The listing builds one solid part. Answer for the finished solid, in the listing's coordinates (mm). Face numbers are marked on the shaded views. Give positions to 0.01 mm unless a question says otherwise; leave off trailing zeros. Write each loop counter-clockwise with the first axis right and the second up, starting at its lowest first coordinate (ties: lowest second). Pieces come first, ordered by that corner, then holes. Notation, with made-up numbers: (-3, 35) - (48, 35) arc R34 cw to (48, 69) - close; hole circle Ø6 at (54, 33). An arc over 180 degrees is marked (long way). Use a Markdown table: item, result. Add a question column.
from build123d import *

# Parameters (mm, degrees)
BOSS_EXTRUDE1_DEPTH     = 6.5
SKETCH2_R               = 27.5
BOSS_EXTRUDE2_DEPTH     = 2.5
CUT_EXTRUDE1_DEPTH      = 8
SKETCH4_W               = 3
SKETCH4_H               = 3
CUT_EXTRUDE2_DEPTH      = 10
SKETCH5_R               = 5
BOSS_EXTRUDE3_DEPTH     = 140
CUT_EXTRUDE3_DEPTH      = 15
MIRROR6_COPY_1_SKETCH_R = 27.5
MIRROR6_COPY_1_DEPTH    = 2.5
MIRROR6_COPY_2_SKETCH_W = 3
MIRROR6_COPY_2_SKETCH_H = 3
MIRROR6_COPY_2_DEPTH    = 10


with BuildPart() as part:
    # Sketch1 → Boss-Extrude1 (new body)
    with BuildSketch(Plane(origin=(0, 0, 0), x_dir=(1, 0, 0), z_dir=(0, 1, 0))):
        with BuildLine():
            ThreePointArc((-1.9, -2.05669638), (-2.8, 0), (-1.9, 2.05669638))
            Line((-1.9, 2.05669638), (-1.9, 5.532856405))
            ThreePointArc((-1.9, 5.532856405), (-5.85, 0), (-1.9, -5.532856405))
            Line((-1.9, -5.532856405), (-1.9, -2.05669638))
        make_face()
        with BuildLine():
            ThreePointArc((-1.9, 2.05669638), (0, 2.8), (1.9, 2.05669638))
            Line((1.9, 2.05669638), (1.9, 5.532856405))
            ThreePointArc((1.9, 5.532856405), (0, 5.85), (-1.9, 5.532856405))
            Line((-1.9, 5.532856405), (-1.9, 2.05669638))
        make_face()
        with BuildLine():
            Line((1.9, 5.532856405), (1.9, 2.05669638))
            ThreePointArc((1.9, 2.05669638), (2.565151068, 1.122497216), (2.8, 0))
            ThreePointArc((2.8, 0), (2.565151068, -1.122497216), (1.9, -2.05669638))
            Line((1.9, -2.05669638), (1.9, -5.532856405))
            ThreePointArc((1.9, -5.532856405), (4.761171074, -3.399080758), (5.85, 0))
            ThreePointArc((5.85, 0), (4.761171074, 3.399080758), (1.9, 5.532856405))
        make_face()
        with BuildLine():
            Line((1.9, -5.532856405), (1.9, -2.05669638))
            ThreePointArc((1.9, -2.05669638), (0, -2.8), (-1.9, -2.05669638))
            Line((-1.9, -2.05669638), (-1.9, -5.532856405))
            ThreePointArc((-1.9, -5.532856405), (0, -5.85), (1.9, -5.532856405))
        make_face()
        with BuildLine():
            Line((-1.9, -2.05669638), (-1.9, 2.05669638))
            ThreePointArc((-1.9, 2.05669638), (-2.8, 0), (-1.9, -2.05669638))
        make_face()
        with BuildLine():
            ThreePointArc((2.8, 0), (2.565151068, 1.122497216), (1.9, 2.05669638))
            Line((1.9, 2.05669638), (1.9, -2.05669638))
            ThreePointArc((1.9, -2.05669638), (2.565151068, -1.122497216), (2.8, 0))
        make_face()
    boss_extrude1 = extrude(amount=BOSS_EXTRUDE1_DEPTH)

    # Sketch2 → Boss-Extrude2 (add)
    with BuildSketch(Plane(origin=(0, 6.5, 0), x_dir=(1, 0, 0), z_dir=(0, 1, 0))):
        with Locations(Location((0, 0, 0), (0, 0, 270))):
            Circle(SKETCH2_R)
    boss_extrude2 = extrude(amount=-BOSS_EXTRUDE2_DEPTH)

    # Sketch3 → Cut-Extrude1 (cut)
    with BuildSketch(Plane.XZ.offset(-4)):
        with BuildLine():
            Line((-1.9, 2.05669638), (-1.9, -2.05669638))
            ThreePointArc((-1.9, -2.05669638), (0, -2.8), (1.9, -2.05669638))
            Line((1.9, -2.05669638), (1.9, 2.05669638))
            ThreePointArc((1.9, 2.05669638), (0, 2.8), (-1.9, 2.05669638))
        make_face()
    cut_extrude1 = extrude(amount=-CUT_EXTRUDE1_DEPTH, mode=Mode.SUBTRACT)

    # Sketch4 → Cut-Extrude2 (cut)
    with BuildSketch(Plane(origin=(0, 6.5, 0), x_dir=(1, 0, 0), z_dir=(0, 1, 0))):
        Polygon((14.299038106, -21.766660498), (15.799038106, -24.36473671), (13.200961894, -25.86473671), (11.700961894, -23.266660498), align=None)
        with Locations((27.5, 0)):
            Rectangle(SKETCH4_W, SKETCH4_H)
        Polygon((-11.700961894, -23.266660498), (-13.200961894, -25.86473671), (-15.799038106, -24.36473671), (-14.299038106, -21.766660498), align=None)
        with Locations((-27.5, 0)):
            Rectangle(SKETCH4_W, SKETCH4_H)
        Polygon((-14.299038106, 21.766660498), (-15.799038106, 24.36473671), (-13.200961894, 25.86473671), (-11.700961894, 23.266660498), align=None)
        Polygon((11.700961894, 23.266660498), (13.200961894, 25.86473671), (15.799038106, 24.36473671), (14.299038106, 21.766660498), align=None)
    cut_extrude2 = extrude(amount=-CUT_EXTRUDE2_DEPTH, mode=Mode.SUBTRACT)

    # Sketch5 → Boss-Extrude3 (add)
    with BuildSketch(Plane(origin=(0, 6.5, 0), x_dir=(1, 0, 0), z_dir=(0, 1, 0))):
        with Locations(Location((0, 0, 0), (0, 0, 270))):
            Circle(SKETCH5_R)
    extrude(amount=BOSS_EXTRUDE3_DEPTH)

    # Mirror1: Boss-Extrude2 across plane
    add(boss_extrude2.mirror(Plane.ZX.offset(76.5)))

    # Mirror2: Boss-Extrude1 across plane
    add(boss_extrude1.mirror(Plane.ZX.offset(76.5)))

    # Mirror3: Boss-Extrude2, Cut-Extrude1, Cut-Extrude2 across plane
    add(boss_extrude2.mirror(Plane.ZX.offset(7.5)))
    add(cut_extrude1.mirror(Plane.ZX.offset(7.5)), mode=Mode.SUBTRACT)
    add(cut_extrude2.mirror(Plane.ZX.offset(7.5)), mode=Mode.SUBTRACT)

    # Sketch6 → Cut-Extrude3 (cut)
    with BuildSketch(Plane.XZ.offset(-11)):
        with BuildLine():
            Line((-1.9, 2.05669638), (-1.9, -2.05669638))
            ThreePointArc((-1.9, -2.05669638), (0, -2.8), (1.9, -2.05669638))
            Line((1.9, -2.05669638), (1.9, 2.05669638))
            ThreePointArc((1.9, 2.05669638), (0, 2.8), (-1.9, 2.05669638))
        make_face()
    extrude(amount=-CUT_EXTRUDE3_DEPTH, mode=Mode.SUBTRACT)

    # Mirror5: Cut-Extrude2 across plane
    add(cut_extrude2.mirror(Plane.ZX.offset(76.5)), mode=Mode.SUBTRACT)

    # Mirror6 copy 1 sketch → Mirror6 copy 1 (add)
    with BuildSketch(Plane(origin=(0, 144.5, 0), x_dir=(1, 0, 0), z_dir=(0, 1, 0))):
        with Locations(Location((0, 0, 0), (0, 0, 270))):
            Circle(MIRROR6_COPY_1_SKETCH_R)
    extrude(amount=-MIRROR6_COPY_1_DEPTH)

    # Mirror6 copy 2 sketch → Mirror6 copy 2 (cut)
    with BuildSketch(Plane(origin=(0, 144.5, 0), x_dir=(1, 0, 0), z_dir=(0, 1, 0))):
        Polygon((14.299038106, -21.766660498), (15.799038106, -24.36473671), (13.200961894, -25.86473671), (11.700961894, -23.266660498), align=None)
        with Locations((27.5, 0)):
            Rectangle(MIRROR6_COPY_2_SKETCH_W, MIRROR6_COPY_2_SKETCH_H)
        Polygon((-11.700961894, -23.266660498), (-13.200961894, -25.86473671), (-15.799038106, -24.36473671), (-14.299038106, -21.766660498), align=None)
        with Locations((-27.5, 0)):
            Rectangle(MIRROR6_COPY_2_SKETCH_W, MIRROR6_COPY_2_SKETCH_H)
        Polygon((-14.299038106, 21.766660498), (-15.799038106, 24.36473671), (-13.200961894, 25.86473671), (-11.700961894, 23.266660498), align=None)
        Polygon((11.700961894, 23.266660498), (13.200961894, 25.86473671), (15.799038106, 24.36473671), (14.299038106, 21.766660498), align=None)
    extrude(amount=-MIRROR6_COPY_2_DEPTH, mode=Mode.SUBTRACT)


solid = part.part
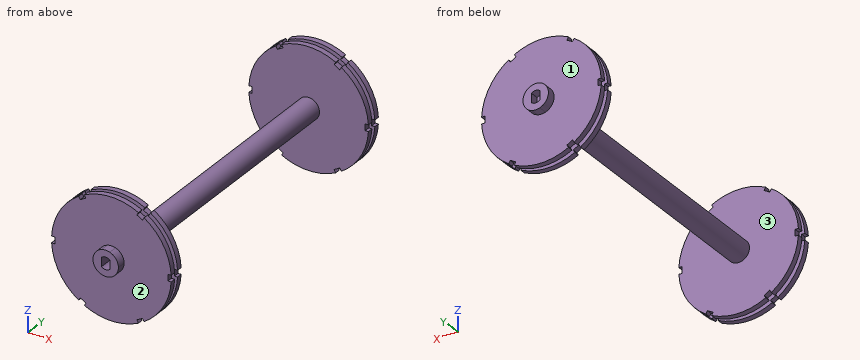
1. The part is cut by section B-B (x = 19). Give the vertices of the cut face in (y, z), and give its area (3 significant figures).
2. Given P1, Ø5, axis at y = 106, z = 6, coming from the +X side; P2, Ø5, axis at x = -5, y = 32, coming from the -Z side; P3, Ø10, axis at y = 136.5, z = 8, coming from the +X side; P4, Ø2, axis at y = 70, z = -7.5, coming from the -X side (1 decimal), each flat-ended and moving along its own axis, determine where each tip first touches the part or whether it passes through.
3. The part is cut by section A-A (z = 9). Give the vertices of the cut face in (x, y), and give its area (3 significant figures).
4. For a pull along Y with two mould halves and no side action, classify the marked faces 1, 2 and 3 as released by +Y, released by -Y, zero draft, split by the parting line, or undercut.
5. The part is cut by section C-C (y = 123). Give the vertices of the cut face in (x, z).
6. Consider L1, parallel to Y at x = 15, z = -20; L2, parallel to X at y = 93, z = -0.5; L3, parallel to X at y = 17, z = 1. Determine where each line is inside the solid, lowest interval first. Write a range as [from, to].
Check values:
| question | item | result |
|---|---|---|
| 1 | outline | (4, -19.88) - (6.5, -19.88) - (6.5, 19.88) - (4, 19.88) - close; (8.5, -19.88) - (11, -19.88) - (11, 19.88) - (8.5, 19.88) - close; (142, -19.88) - (144.5, -19.88) - (144.5, 19.88) - (142, 19.88) - close; (146.5, -19.88) - (149, -19.88) - (149, 19.88) - (146.5, 19.88) - close |
| 1 | area | 398 mm2 |
| 2 | P1 | stops at x = 3.57 |
| 2 | P2 | stops at z = -4.33 |
| 2 | P3 | stops at x = 4 |
| 2 | P4 | passes through |
| 3 | outline | (-25.99, 4) - (25.99, 4) - (25.99, 6.5) - (-25.99, 6.5) - close; (-25.99, 8.5) - (25.99, 8.5) - (25.99, 11) - (-25.99, 11) - close; (-25.99, 142) - (25.99, 142) - (25.99, 144.5) - (-25.99, 144.5) - close; (-25.99, 146.5) - (25.99, 146.5) - (25.99, 149) - (-25.99, 149) - close |
| 3 | area | 520 mm2 |
| 4 | face 1 | released by +Y |
| 4 | face 2 | released by -Y |
| 4 | face 3 | undercut |
| 5 | outline | circle Ø10 at (0, 0) |
| 6 | L1 | y = [4, 6.5], [8.5, 11], [142, 144.5], [146.5, 149] |
| 6 | L2 | x = [-4.97, 4.97] |
| 6 | L3 | x = [-4.9, -1.9], [1.9, 4.9] |
